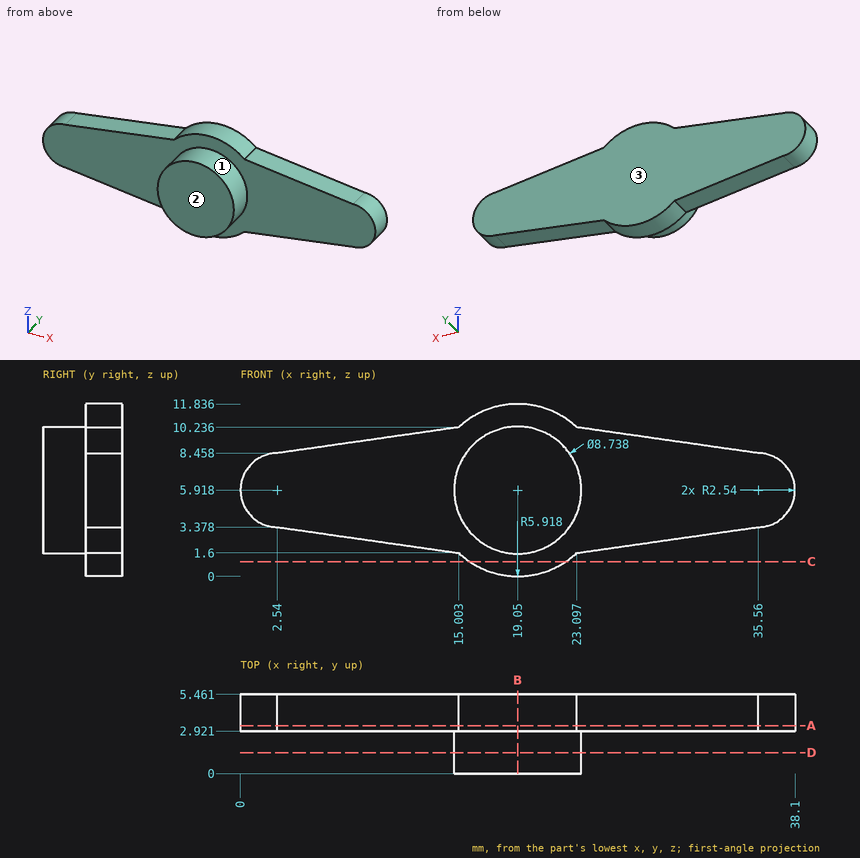
Input: dimensioned drawing with shaded views. Units: mm. Origin: part minimum x, y, z. Coordinates: 2 decimals unless noted, no trailing zeros. Order: outer loops, then holes, each group sorted by start corner. A loop starts at its lowest first (then second) coordinate and runs counter-clockwise, first axis right, second up. Notation, with made-up numbers: (-34.75, 65) - (22.25, 65) arc R25 cw to (22.25, 83) - close; hole circle Ø3 at (59, 82). An arc over 180 degrees is marked (long way). Return JSON: item names as keys, results as strings. Group by question number.
1. Cut plane B-B (x = 19.05). Output: boundary loops of the cut face in (y, z).
2. Cut plane C-C (z = 1). Output: boundary loops of the cut face in (x, y), plus the area to 3 significant figures.
3. Pull-direction query (Y, two-part tool) for the marked faces 1, 2 and 3; classes: pulls with the +Y half, pulls with the -Y half, needs draft (parallel to the pull), parting line crosses it, or undercut.
4. Cut plane A-A (y = 3.3). Output: boundary loops of the cut face in (x, z), plus the area to 3 significant figures.
5. Material intervals for line 1 along Y through (x, z) = (22.5, 9.5); line 2 along X through (y, z) = (3.35, 1.5) (1 decimal); line 3 along X through (y, z) = (0.3, 8), sorted ascending. Write a range as [from, to].
6. Cut plane D-D (y = 1.45). Output: boundary loops of the cut face in (x, z).
7. Pin query (flat end, axial travel): pin 1 (6 mm diameter, centred on x = 14, z = 3.5, fed in from -Y); pin 2 (5 mm diameter, centred on x = 30, z = 4.5, fed in from -Y). Return the tip coordinate at first contact, or that it passes through.
Resolved:
{
 "1": {"outline": "(0, 1.55) - (2.92, 1.55) - (2.92, 0) - (5.46, 0) - (5.46, 11.84) - (2.92, 11.84) - (2.92, 10.29) - (0, 10.29) - close"},
 "2": {"outline": "(15.76, 2.92) - (22.34, 2.92) - (22.34, 5.46) - (15.76, 5.46) - close", "area": "16.7 mm²"},
 "3": {"face 1": "needs draft", "face 2": "pulls with the -Y half", "face 3": "pulls with the +Y half"},
 "4": {"outline": "(2.54, 3.38) - (15, 1.6) arc R5.92 ccw to (23.1, 1.6) - (35.56, 3.38) arc R2.54 ccw to (35.56, 8.46) - (23.1, 10.24) arc R5.92 ccw to (15, 10.24) - (2.54, 8.46) arc R2.54 ccw to start", "area": "279 mm²"},
 "5": {"line 1": "y = [2.92, 5.46]", "line 2": "x = [15.1, 23]", "line 3": "x = [15.21, 22.89]"},
 "6": {"outline": "circle Ø8.74 at (19.05, 5.92)"},
 "7": {"pin 1": "stops at y = 0", "pin 2": "stops at y = 2.92"}
}
